Autodesk Inventor part; units mm, degrees
ref_plane "YZ Plane" through (0, 0, 0) normal (1, 0, 0) x (0, 1, 0)
ref_plane "XZ Plane" through (0, 0, 0) normal (0, 1, 0) x (-1, 0, 0)
ref_plane "XY Plane" through (0, 0, 0) normal (0, 0, 1) x (1, 0, 0)
sketch "スケッチ1" plane through (0, 0, 0) normal (0, 1, 0) x (-1, 0, 0)
  line L0 (2, 0) -> (25, 0)
  line L1 (27, -2) -> (27, -40)
  line L2 (25, -42) -> (2, -42)
  line L3 (0, -40) -> (0, -2)
  arc A0 (27, -2) -> (25, 0) centre (25, -2) ccw
  arc A1 (25, -42) -> (27, -40) centre (25, -40) ccw
  arc A2 (2, 0) -> (0, -2) centre (2, -2) ccw
  arc A3 (0, -40) -> (2, -42) centre (2, -40) ccw
  point P0 (0, 0)
  point P1 (27, -42)
  point P2 (27, 0)
  point P3 (0, -42)
  dimension "d0" = 27
  dimension "d1" = 42
  dimension "d2" = 2
extrude "押し出し1" add sketch "スケッチ1" along normal blind 2
sketch "スケッチ2" plane through (0, 2, 0) normal (0, 1, 0) x (1, 0, 0)
  line L0 (-27, 40) -> (-27, 2)
  line L1 (0, 2) -> (0, 40)
  line L2 (-2, 42) -> (-25, 42)
  line L3 (-25, 0) -> (-2, 0)
  point P0 (0, 0)
  point P1 (-21, 39)
  point P2 (-6, 39)
  point P3 (-21, 3)
  point P4 (-6, 3)
  dimension "d5" = 6
  dimension "d6" = 6
  dimension "d7" = 6
  dimension "d8" = 6
  dimension "d9" = 3
  dimension "d10" = 3
  dimension "d11" = 3
  dimension "d12" = 3
hole "穴1" at (-21, 2, -39) at (-6, 2, -39) at (-21, 2, -3) at (-6, 2, -3) direction (0, -1, 0) diameter 3.1 end through all
sketch "スケッチ3" plane through (0, 2, 0) normal (0, 1, 0) x (1, 0, 0)
  line L0 (-27, 40) -> (-27, 2)
  line L1 (-27, 34.5) -> (0, 34.5)
  line L2 (0, 34.5) -> (0, 7.5)
  line L3 (0, 7.5) -> (-27, 7.5)
  line L4 (-27, 7.5) -> (-27, 34.5)
  line L5 (0, 2) -> (0, 40)
  circle A0 centre (-13.5, 3) radius 2.75
  circle A1 centre (-13.5, 39) radius 2.75
  arc A2 (-20.75, 34.5) -> (-16.25, 39) centre (-20.75, 39) ccw
  arc A3 (-10.75, 39) -> (-6.25, 34.5) centre (-6.25, 39) ccw
  line L6 (-16.25, 3) -> (-20.75, 3)
  line L7 (-10.75, 3) -> (-6.25, 3)
  arc A4 (-16.25, 3) -> (-20.75, 7.5) centre (-20.75, 3) ccw
  arc A5 (-6.25, 7.5) -> (-10.75, 3) centre (-6.25, 3) ccw
  point P0 (0, 0)
  point P1 (0, 21)
  point P2 (0, 21)
  dimension "d20" = 27
  dimension "d21" = 27
  dimension "d22" = 0
  dimension "d23" = 5.5
  dimension "d24" = 5.5
  dimension "d25" = 4.5
  dimension "d27" = 4.5
  dimension "d29" = 4.5
  dimension "d30" = 4.5
extrude "押し出し2" add sketch "スケッチ3" along normal blind 12
sketch "スケッチ4" plane through (0, 0, -2) normal (1, 0, 0) x (0, 0, -1)
  line L0 (32.5, 14) -> (5.5, 14)
  circle A0 centre (19, 14) radius 12
  point P0 (-2, 0)
  point P1 (7, 14)
  point P2 (31, 14)
  dimension "d33" = 24
extrude "押し出し3" cut sketch "スケッチ4" against normal through all contours A0 L0 picked at (15.4582, 12.1411)
sketch "スケッチ5" plane through (0, 14, 0) normal (0, 1, 0) x (1, 0, 0)
  arc A0 (-10.75, 39) -> (-16.25, 39) centre (-13.5, 39) ccw
  arc A1 (-16.25, 3) -> (-10.75, 3) centre (-13.5, 3) ccw
  point P0 (0, 0)
hole "穴2" at (-13.5, 14, -39) at (-13.5, 14, -3) direction (0, -1, 0) diameter 2.8 end through all
properties part number "daisen_moto_parts1"
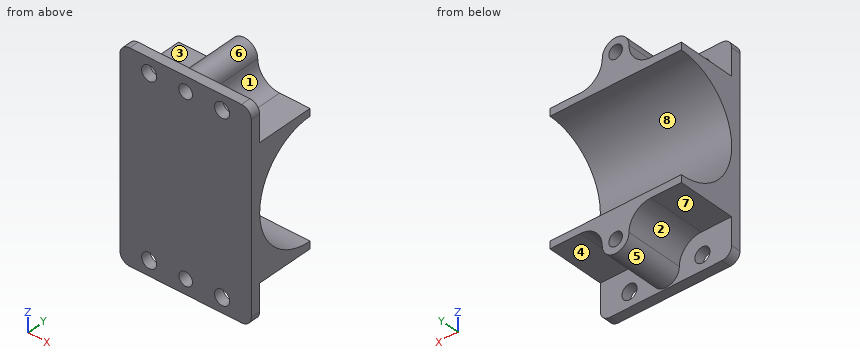
Geometry check sheet. Reference: the model listing, model coordinates, mm. Face numbers are marked on the shaded views. A direction names the side the tool comes from. Give positions to 0.01 mm unless a question says otherwise; leave off trailing zeros. Order: outer loops, then holes, each group sorted by start corner. A loop starts at its lowest first (then second) coordinate and runs counter-clockwise, first axis right, second up. Notation, with made-up numbers: (-36, -30.75) - (-2, -30.75) arc R20 cw to (-2, -26.75) - close; hole circle Ø8 at (17, -39.5). An arc over 180 degrees is marked (long way). Answer in a Markdown table with one row per item. Add a question column.
Q1. Cross-section at B-B, the plane x = -5.5. Enter the section's corners in (y, z), then the cut area to 3 significant figures.
Q2. Cross-section at A-A, the plane y = 3.5. Enter the section's corners in (x, z), then the cut area to 3 significant figures.
Q3. Tool access check on the marked faces 1, 2, 3, 4 and 5. Record the directions out of +Z, -Z, +X, -X, +Y, -Y that give a thin tool (end or side, any length) a straight path to the whole face; none if there is none.
Q4. Mould release check, pull along Z, two halves, no side actions. Record for the marked faces 6, 7 and 8: pulls with the +Z half, pulls with the -Z half, needs draft (parallel to the pull), parting line crosses it, or undercut.
Q5. Material ranges on probe 1 along Z at (x, y) = (-6, 1.45); probe 2 along X at (y, z) = (1.3, -3); probe 3 along X at (y, z) = (6.5, -3), recorded low to high. Write a range as from..to.
Q6. Gauge pin test, flat ends, axial feed: pin 1 (3 mm diameter, centred on x = -22.5, y = 5.5, fed in from -Z); pin 2 (5 mm diameter, centred on x = -4.5, y = 9, fed in from +Z); pin 3 (2.5 mm diameter, centred on x = -13.5, z = -39, fed in from +Y); pin 4 (3 mm diameter, centred on x = -25.5, y = 10, fed in from +Z). Record the tip position at first contact, or that the pin passes through.
Q7. Cross-section at C-C, the plane y = 8.75. Enter the section's corners in (x, z).
Q8. Cross-section at D-D, the plane z = -7. Enter the section's corners in (x, y).
Check values:
| question | item | result |
|---|---|---|
| 1 | outline | (0, -42) - (2, -42) - (2, -40.47) - (0, -40.47) - close; (0, -37.53) - (2, -37.53) - (2, -34.5) - (14, -34.5) - (14, -33) arc R12 cw to (14, -9) - (14, -7.5) - (2, -7.5) - (2, -4.47) - (0, -4.47) - close; (0, -1.53) - (2, -1.53) - (2, 0) - (0, 0) - close |
| 1 | area | 170 mm^2 |
| 2 | outline | (-27, -34.5) - (-20.75, -34.5) arc R4.5 cw to (-16.25, -39) arc R2.75 ccw to (-10.75, -39) arc R4.5 cw to (-6.25, -34.5) - (0, -34.5) - (0, -26.81) - (-27, -26.81) - close; (-27, -15.19) - (0, -15.19) - (0, -7.5) - (-6.25, -7.5) arc R4.5 cw to (-10.75, -3) arc R2.75 ccw to (-16.25, -3) arc R4.5 cw to (-20.75, -7.5) - (-27, -7.5) - close; hole circle Ø2.8 at (-13.5, -39); hole circle Ø2.8 at (-13.5, -3) |
| 2 | area | 494 mm^2 |
| 3 | face 1 | +Z, +X, +Y |
| 3 | face 2 | -Z, -X, +Y |
| 3 | face 3 | +Z, -X, +Y |
| 3 | face 4 | -Z, +X, +Y |
| 3 | face 5 | -Z, +Y |
| 4 | face 6 | pulls with the +Z half |
| 4 | face 7 | pulls with the -Z half |
| 4 | face 8 | undercut |
| 5 | probe 1 | z = -42..-40.55, -37.45..-4.55, -1.45..0 |
| 5 | probe 2 | x = -27..-22.55, -19.45..-14.9, -12.1..-7.55, -4.45..0 |
| 5 | probe 3 | x = -16.25..-14.9, -12.1..-10.75 |
| 6 | pin 1 | stops at z = -34.5 |
| 6 | pin 2 | stops at z = -7.44 |
| 6 | pin 3 | passes through |
| 6 | pin 4 | stops at z = -7.5 |
| 7 | outline | (-27, -34.5) - (-20.75, -34.5) arc R4.5 cw to (-16.25, -39) arc R2.75 ccw to (-10.75, -39) arc R4.5 cw to (-6.25, -34.5) - (0, -34.5) - (0, -31.79) - (-27, -31.79) - close; (-27, -10.21) - (0, -10.21) - (0, -7.5) - (-6.25, -7.5) arc R4.5 cw to (-10.75, -3) arc R2.75 ccw to (-16.25, -3) arc R4.5 cw to (-20.75, -7.5) - (-27, -7.5) - close; hole circle Ø2.8 at (-13.5, -39); hole circle Ø2.8 at (-13.5, -3) |
| 8 | outline | (-27, 0) - (0, 0) - (0, 2) - (-8.31, 2) - (-8.31, 14) - (-18.69, 14) - (-18.69, 2) - (-27, 2) - close |
